Design review of the part built by this model. Coordinates are the model's own, in mm. A direction names the side the tool comes from. Give positions to 0.01 mm unless a question says otherwise; leave off trailing zeros. Loops run counter-clockwise (first coordinate to the right, second up) from the corner with the lowest first, then second, coordinate; pieces in that order, holes last. Notation, with made-up numbers: M 25.5,9.25 L 70.5,9.25 A18 ccw 70.5,22.25 Z; hole C -32.5,8.5 d2. An arc over 180 degrees is marked long. Answer as CSV lines item,"result".
```python
from build123d import *

# Parameters (mm, degrees)
SKETCH1_W             = 45
SKETCH1_H             = 45
BOSS_EXTRUDE1_DEPTH   = 17.5
CUT_EXTRUDE1_REACH    = 55.268
SKETCH2_R             = 12.8397
SKETCH3_R             = 12.8397
CUT_EXTRUDE2_DEPTH    = 54.268189382
CUT_EXTRUDE3_DEPTH    = 13.2
CUT_EXTRUDE4_DEPTH    = 31.819805153
M3_TAPPED_HOLE1_D     = 2.5
M3_TAPPED_HOLE1_DEPTH = 6.5
M3_TAPPED_HOLE1_TIP   = 0.751075774
M3_TAPPED_HOLE2_D     = 2.5
M3_TAPPED_HOLE2_DEPTH = 5.5
M3_TAPPED_HOLE2_TIP   = 0.751075774
M2_TAPPED_HOLE1_D     = 1.6
M2_TAPPED_HOLE1_DEPTH = 5.2
M2_TAPPED_HOLE1_TIP   = 0.480688495


# Read off the part's stored shape, not the designer's step: Cut-Extrude4
with BuildPart() as part:
    # Sketch1 → Boss-Extrude1 (new, symmetric)
    with BuildSketch(Plane(origin=(0, 0, 0), x_dir=(1, 0, 0), z_dir=(0, 1, 0))):
        Rectangle(SKETCH1_W, SKETCH1_H)
    extrude(amount=BOSS_EXTRUDE1_DEPTH, both=True)

    # Sketch2 → Cut-Extrude1 (cut, up to next)
    with BuildSketch(Plane(origin=(22.5, 0, 0), x_dir=(0, 0, -1), z_dir=(1, 0, 0)), mode=Mode.PRIVATE) as cut_extrude1_sk1:
        Circle(SKETCH2_R)
    cut_extrude1_tool1 = extrude(cut_extrude1_sk1.sketch, amount=-CUT_EXTRUDE1_REACH, mode=Mode.PRIVATE) & part.part
    add(cut_extrude1_tool1.solids().sort_by_distance((22.5, 0, 0))[0], mode=Mode.SUBTRACT)

    # Sketch3 → Cut-Extrude2 (cut, through all)
    with BuildSketch(Plane(origin=(0, 0, -22.5), x_dir=(-1, 0, 0), z_dir=(0, 0, -1))):
        Circle(SKETCH3_R)
    extrude(amount=-CUT_EXTRUDE2_DEPTH, mode=Mode.SUBTRACT)

    # Sketch5 → Cut-Extrude3 (cut, symmetric)
    with BuildSketch(Plane(origin=(0, 0, 0), x_dir=(1, 0, 0), z_dir=(0, 1, 0))):
        Polygon((-12.727922061, -12.727922061), (12.727922061, 12.727922061), (11.914749263, 13.54109486), (-13.54109486, -11.914749263), align=None)
    extrude(amount=CUT_EXTRUDE3_DEPTH, both=True, mode=Mode.SUBTRACT)

    # Cut-Extrude4 outline → Cut-Extrude4 (cut)
    with BuildSketch(Plane(origin=(0, 0, 0), x_dir=(-0.7071067811865486, 0, 0.7071067811865465), z_dir=(-0.7071067811865465, 0, -0.7071067811865486))):
        with BuildLine():
            ThreePointArc((-14, 13.2), (-16, 15.2), (-18, 13.2))
            Line((-18, 13.2), (-18, -13.2))
            ThreePointArc((-18, -13.2), (-16, -15.2), (-14, -13.2))
            Line((-14, -13.2), (14, -13.2))
            ThreePointArc((14, -13.2), (16, -15.2), (18, -13.2))
            Line((18, -13.2), (18, 13.2))
            ThreePointArc((18, 13.2), (16, 15.2), (14, 13.2))
            Line((14, 13.2), (-14, 13.2))
        make_face()
    extrude(amount=CUT_EXTRUDE4_DEPTH, mode=Mode.SUBTRACT)

    # M3 Tapped Hole1
    with Locations(Plane.XY.offset(22.5)):
        with Locations((-10, -13.5), (10, -13.5), (10, 13.5), (-10, 13.5)):
            Hole(M3_TAPPED_HOLE1_D / 2, depth=M3_TAPPED_HOLE1_DEPTH)
            with Locations((0, 0, -(M3_TAPPED_HOLE1_DEPTH + M3_TAPPED_HOLE1_TIP / 2))):  # 118° drill point
                Cone(0, M3_TAPPED_HOLE1_D / 2, M3_TAPPED_HOLE1_TIP, mode=Mode.SUBTRACT)

    # M3 Tapped Hole2
    with Locations(Plane(origin=(0, 0, -22.5), x_dir=(-1, 0, 0), z_dir=(0, 0, -1))):
        with Locations((-10, 13.5), (-10, -13.5)):
            Hole(M3_TAPPED_HOLE2_D / 2, depth=M3_TAPPED_HOLE2_DEPTH)
            with Locations((0, 0, -(M3_TAPPED_HOLE2_DEPTH + M3_TAPPED_HOLE2_TIP / 2))):  # 118° drill point
                Cone(0, M3_TAPPED_HOLE2_D / 2, M3_TAPPED_HOLE2_TIP, mode=Mode.SUBTRACT)

    # M2 Tapped Hole1
    with Locations(Plane(origin=(0, 0, 0), x_dir=(-0.7071067811865486, 0, 0.7071067811865465), z_dir=(-0.7071067811865465, 0, -0.7071067811865486))):
        with Locations((-16, -13.75), (-16, 13.75), (16, 13.75), (16, -13.75)):
            Hole(M2_TAPPED_HOLE1_D / 2, depth=M2_TAPPED_HOLE1_DEPTH)
            with Locations((0, 0, -(M2_TAPPED_HOLE1_DEPTH + M2_TAPPED_HOLE1_TIP / 2))):  # 118° drill point
                Cone(0, M2_TAPPED_HOLE1_D / 2, M2_TAPPED_HOLE1_TIP, mode=Mode.SUBTRACT)


solid = part.part
```
1. The part is to be moulded in two halves that separate along Z. For faces 1 (the cylindrical face through (-17.6, 15.2, 5.1)), 2 (the cylindrical face through (-9.523, 14.543, 13.252)), 3 (the flat face through (-10.3, 8, 22.5)), 4 (the cylindrical face through (-9.079, -12.655, 19.204)), say which applies: pulls with the +Z half, pulls with the -Z half, needs draft (parallel to the pull), parting line crosses it, or undercut.
Answer block:
face 1,"undercut"
face 2,"undercut"
face 3,"pulls with the +Z half"
face 4,"needs draft"
2. To check wall thickness, follow L1, parallel to X at y = -13.5, z = 18.75; L2, parallel to X at y = 3, z = 15; L3, parallel to Y at x = 10, z = 19. State the ranges of each line that lie inside material, in increasing order. Write a range as [from, to].
Answer block:
L1,"[-22.5, -11.25], [-8.75, 8.75], [11.25, 22.5]"
L2,"[-22.5, -12.48], [12.48, 22.5]"
L3,"[-17.5, -14.75], [-12.25, -8.05], [8.05, 12.25], [14.75, 17.5]"
3. For faces 5 (the flat face through (1, 13, -1)), 6 (the cylindrical face through (-18.631, 0.241, 12.837)), 7 (the cylindrical face through (-9.079, 14.345, 19.204)), 8 (the cylindrical face through (9.079, 14.345, -19.712)), list the 3-axis set-ups (+Z, -Z, +X, -X, +Y, -Y) from which the entire face can be reached by the end or side of a thin tool; tool diameter is ignored.
Answer block:
face 5,"none"
face 6,"-Z, +X, -X"
face 7,"+Z"
face 8,"-Z"
4. We need section B-B, the plane y = -3.5. Write out the cut boundary in (x, z), plus the area to 3 significant figures.
Answer block:
outline,"M -22.5,12.35 L -13.1,12.35 L -12.73,12.73 L -12.35,12.35 L -12.35,22.5 L -22.5,22.5 Z; M 12.35,-22.5 L 22.5,-22.5 L 22.5,-12.35 L 12.35,-12.35 L 12.73,-12.73 L 12.35,-13.1 Z; M 12.35,12.35 L 22.5,12.35 L 22.5,22.5 L 12.35,22.5 Z"
area,"309 mm²"
5. We need section C-C, the plane x = 17. Write out the cut boundary in (y, z), plus the area to 3 significant figures.
Answer block:
outline,"M -17.5,-22.5 L 17.5,-22.5 L 17.5,22.5 L -17.5,22.5 Z; hole C 0,0 d25.68"
area,"1,060 mm²"
6. We need section A-A, the plane z = 18.5. Write out the cut boundary in (x, y), plus the area to 3 significant figures.
Answer block:
outline,"M -22.5,-17.5 L 22.5,-17.5 L 22.5,17.5 L -22.5,17.5 Z; hole C 0,0 d25.68; hole C -10,-13.5 d2.5; hole C -10,13.5 d2.5; hole C 10,-13.5 d2.5; hole C 10,13.5 d2.5"
area,"1,040 mm²"
7. For P1, Ø2, axis at x = 10, y = 13.5, coming from the +Z side; P2, Ø3, axis at y = -9.5, z = -6.5, coming from the -X side; P3, Ø2, axis at y = -3, z = -12, coming from the -X side, all flat-tipped, find the tip position at first contact; note any pin that passes through.
Answer block:
P1,"z = 15.85"
P2,"x = 6.63"
P3,"x = 12.21"
8. We need section D-D, the plane y = 4. Write out the cut boundary in (x, z).
Answer block:
outline,"M -22.5,12.2 L -13.26,12.2 L -12.73,12.73 L -12.2,12.2 L -12.2,22.5 L -22.5,22.5 Z; M 12.2,-22.5 L 22.5,-22.5 L 22.5,-12.2 L 12.2,-12.2 L 12.73,-12.73 L 12.2,-13.26 Z; M 12.2,12.2 L 22.5,12.2 L 22.5,22.5 L 12.2,22.5 Z"
